Input: part model. Units: mm. Frame: model coordinates. Give positions to 0.01 mm unless a question says otherwise; leave off trailing zeros. Order: outer loops, then holes, each group sorted by start corner. A loop starts at its lowest first (then second) coordinate and runs counter-clockwise, first axis right, second up.
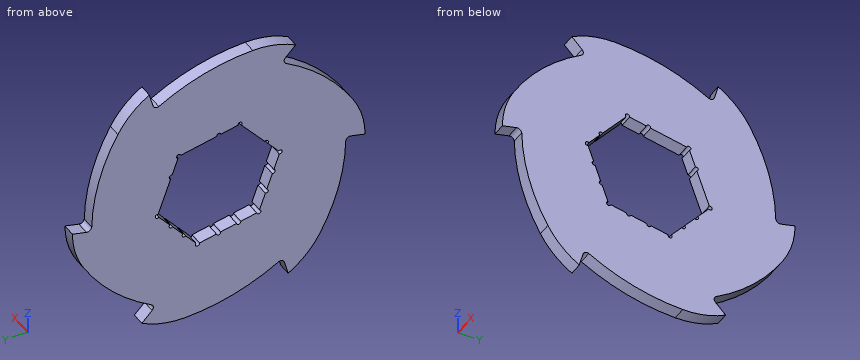
```python
from build123d import *

# Parameters (mm, degrees)
SKETCH1_R                = 59
EXTRUDE1_DEPTH           = 3
EXTRUDE2_DEPTH           = 3
CIRPATTERN1_COUNT        = 6
F_2_0_2_DIAMETER_HOLE1_D = 2
F_2_0_2_DIAMETER_HOLE3_D = 2
F_2_0_2_DIAMETER_HOLE4_D = 2
CIRPATTERN2_COUNT        = 6
CIRPATTERN3_COUNT        = 3
CIRPATTERN3_ANGLE        = 120


with BuildPart() as part:
    # Sketch1 → Extrude1 (new, symmetric)
    with BuildSketch(Plane(origin=(0, 0, 0), x_dir=(0, 0, -1), z_dir=(1, 0, 0))):
        Circle(SKETCH1_R)
        Polygon((27.180842557, 9.893017633), (5.022816688, 28.485808967), (-22.158025869, 18.592791334), (-27.180842557, -9.893017633), (-5.022816688, -28.485808967), (22.158025869, -18.592791334), align=None, mode=Mode.SUBTRACT)
    extrude(amount=EXTRUDE1_DEPTH, both=True)

    # Sketch2 → Extrude2 (add, symmetric)
    with BuildSketch(Plane(origin=(0, 0, 0), x_dir=(0, 0, -1), z_dir=(1, 0, 0))):
        with BuildLine():
            Line((-2, 67.961805723), (-0.262709442, 61.478149092))
            ThreePointArc((-0.262709442, 61.478149092), (-0.58620663, 59.77173183), (-2.122608272, 58.961805723))
            ThreePointArc((-2.122608272, 58.961805723), (28.679663449, 51.560419941), (51.21368579, 29.294340542))
            ThreePointArc((51.21368579, 29.294340542), (36.791707484, 48.186627241), (17.927108603, 62.644803614))
            ThreePointArc((17.927108603, 62.644803614), (8.312130826, 66.609702921), (-2, 67.961805723))
        make_face()
    extrude2 = extrude(amount=EXTRUDE2_DEPTH, both=True)

    # CirPattern1: Extrude2 ×6 about axis
    cirpattern1_axis = Axis((0, 0, 0), (1, 0, 0))
    for i in range(1, CIRPATTERN1_COUNT):
        add(extrude2.rotate(cirpattern1_axis, i * 360 / CIRPATTERN1_COUNT))

    # Ø2.0 (2) Diameter Hole1 (through all)
    with Locations(Plane(origin=(3, 0, 0), x_dir=(0, 0, -1), z_dir=(1, 0, 0))):
        with Locations((5.022816688, 28.485808967), (27.180842557, 9.893017633), (22.158025869, -18.592791334), (-5.022816688, -28.485808967), (-27.180842557, -9.893017633), (-22.158025869, 18.592791334)):
            Hole(F_2_0_2_DIAMETER_HOLE1_D / 2)

    # Ø2.0 (2) Diameter Hole3 (through all)
    with Locations(Plane(origin=(3, 0, 0), x_dir=(0, 0, -1), z_dir=(1, 0, 0))):
        with Locations((12.664173459, 22.073949319)):
            f_2_0_2_diameter_hole3 = Hole(F_2_0_2_DIAMETER_HOLE3_D / 2)

    # Ø2.0 (2) Diameter Hole4 (through all)
    with Locations(Plane(origin=(3, 0, 0), x_dir=(0, 0, -1), z_dir=(1, 0, 0))):
        with Locations((19.922508008, 15.983483476)):
            f_2_0_2_diameter_hole4 = Hole(F_2_0_2_DIAMETER_HOLE4_D / 2)

    # CirPattern2: Ø2.0 (2) Diameter Hole3 ×6 about axis
    cirpattern2_axis = Axis((0, 0, 0), (1, 0, 0))
    for i in range(1, CIRPATTERN2_COUNT):
        add(f_2_0_2_diameter_hole3.rotate(cirpattern2_axis, i * 360 / CIRPATTERN2_COUNT), mode=Mode.SUBTRACT)

    # CirPattern3: Ø2.0 (2) Diameter Hole4 ×3 about axis
    cirpattern3_axis = Axis((0, 0, 0), (-1, 0, 0))
    for i in range(1, CIRPATTERN3_COUNT):
        add(f_2_0_2_diameter_hole4.rotate(cirpattern3_axis, i * CIRPATTERN3_ANGLE / (CIRPATTERN3_COUNT - 1)), mode=Mode.SUBTRACT)


solid = part.part
```
1) First-contact query: P1, Ø1.5, axis at x = 0, z = -38, coming from the -Y side; P2, Ø3, axis at x = 0.5, y = -41.5, coming from the +Z side. Flat tips, straight axial feed; report the tip coordinate or a pass-through.
2) Line query: probe 1 along Y at (x, z) = (2.4, -13.5); probe 2 along Y at (x, z) = (-2.2, -9); probe 3 along Y at (x, z) = (0.8, 10). Output: solid intervals per line, ascending.
3) Cut plane B-B (z = -16). Return the cut outline in (x, y).
4) Cut plane D-D (y = -45). Return the cut outline in (x, z), then the cut area to 3 significant figures.
5) Cut plane C-C (z = -47). Return the cut outline in (x, y).
6) Cut plane A-A (y = 34). Return the cut outline in (x, z), then the cut area to 3 significant figures.
Geometry says:
1. P1: stops at y = -50.99
1. P2: stops at z = 44.03
2. probe 1: y = -58 to -22.7, 21.37 to 21.52, 22.62 to 64.84
2. probe 2: y = -58.56 to -23.38, 25.15 to 66.42
2. probe 3: y = -66.12 to -24.31, 23.02 to 58.46
3. outline: (-3, -57.59) - (3, -57.59) - (3, -20.83) - (-3, -20.83) - close; (-3, 19.27) - (3, 19.27) - (3, 63.68) - (-3, 63.68) - close
4. outline: (-3, -48.18) - (3, -48.18) - (3, 39.82) - (-3, 39.82) - close
4. area: 528 mm2
5. outline: (-3, -45.8) - (3, -45.8) - (3, 35.96) - (-3, 35.96) - close
6. outline: (-3, -58.79) - (3, -58.79) - (3, -56.14) - (-3, -56.14) - close; (-3, -48.33) - (3, -48.33) - (3, 58.78) - (-3, 58.78) - close
6. area: 659 mm2
